Answer from the drawing. Dimensions are ordinates in mm from the lowest x, y and z of the part. Round coordinates to 2 decimals unless told otherwise and drop trailing zeros. Loops run counter-clockwise (first coordinate to the right, second up) from the corner with the lowest first, then second, coordinate; pieces in that order, holes last.
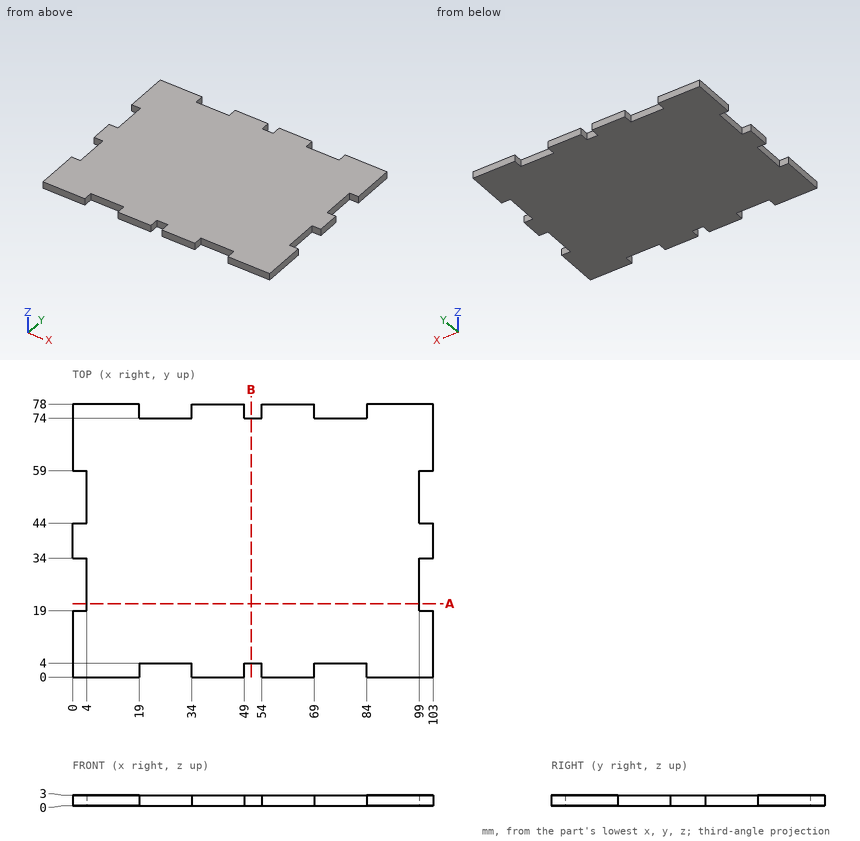
1. Given pin 1 (1.5 mm diameter, centred on x = 72, z = 2, fed in from +Y); pin 2 (0.9 mm diameter, centred on y = 48.5, z = 2, fed in from -X); pin 3 (1.5 mm diameter, centred on y = 47, z = 0.5, fed in from +X), each flat-ended and moving along its own axis, determine where each tip first touches the part or whether it passes through.
Answer key:
pin 1: stops at y = 74
pin 2: stops at x = 4
pin 3: stops at x = 99
2. Find section B-B (x = 51). Write down the section's boundary in (y, z), then the cut area to 3 significant figures.
Answer key:
outline: (4, 0) - (74, 0) - (74, 3) - (4, 3) - close
area: 210 mm2
3. Consider probe 1 along Y at (x, z) = (70, 2.2); probe 2 along X at (y, z) = (47, 1). Determine where each line is inside the solid, lowest interval first.
Answer key:
probe 1: y = 4 to 74
probe 2: x = 4 to 99
4. Find section A-A (y = 21). Write down the section's boundary in (x, z), then the cut area to 3 significant figures.
Answer key:
outline: (4, 0) - (99, 0) - (99, 3) - (4, 3) - close
area: 285 mm2
